```python
from build123d import *

# Parameters (mm, degrees)
PAD_DEPTH       = 18
SKETCH001_R     = 6
POCKET_DEPTH    = 18
SKETCH006_R     = 12.75
POCKET003_DEPTH = 2.4


with BuildPart() as part:
    # Sketch → Pad (new body)
    with BuildSketch(Plane.XY):
        with BuildLine():
            Line((-360, 420), (360, 420))
            Line((360, 420), (360, 36))
            ThreePointArc((324, 0), (349.455844, 10.544156), (360, 36))
            Line((324, 0), (-324, 0))
            ThreePointArc((-360, 36), (-349.455844, 10.544156), (-324, 0))
            Line((-360, 36), (-360, 420))
        make_face()
    extrude(amount=PAD_DEPTH)

    # Sketch001 → Pocket (cut)
    with BuildSketch(Plane.XY.offset(18)):
        with Locations((-85, 125)):
            Circle(SKETCH001_R)
        with Locations((-85, 295)):
            Circle(SKETCH001_R)
        with Locations((85, 295)):
            Circle(SKETCH001_R)
        with Locations((85, 125)):
            Circle(SKETCH001_R)
        with BuildLine():
            ThreePointArc((-274, 253), (-290, 269), (-306, 253))
            Line((-306, 253), (-306, 73))
            ThreePointArc((-306, 73), (-290, 57), (-274, 73))
            Line((-274, 73), (-274, 253))
        make_face()
        with BuildLine():
            ThreePointArc((-136.333333, 253), (-152.333333, 269), (-168.333333, 253))
            Line((-168.333333, 253), (-168.333333, 73))
            ThreePointArc((-168.333333, 73), (-152.333333, 57), (-136.333333, 73))
            Line((-136.333333, 73), (-136.333333, 253))
        make_face()
        with BuildLine():
            ThreePointArc((306, 253), (290, 269), (274, 253))
            Line((274, 73), (274, 253))
            ThreePointArc((274, 73), (290, 57), (306, 73))
            Line((306, 253), (306, 73))
        make_face()
        with BuildLine():
            ThreePointArc((168.333333, 253), (152.333333, 269), (136.333333, 253))
            Line((136.333333, 73), (136.333333, 253))
            ThreePointArc((136.333333, 73), (152.333333, 57), (168.333333, 73))
            Line((168.333333, 253), (168.333333, 73))
        make_face()
        with BuildLine():
            Line((-27, 324), (27, 324))
            ThreePointArc((39, 312), (35.485281, 320.485281), (27, 324))
            Line((39, 312), (39, 148))
            ThreePointArc((27, 136), (35.485281, 139.514719), (39, 148))
            Line((27, 136), (-27, 136))
            ThreePointArc((-39, 148), (-35.485281, 139.514719), (-27, 136))
            Line((-39, 148), (-39, 312))
            ThreePointArc((-27, 324), (-35.485281, 320.485281), (-39, 312))
        make_face()
    extrude(amount=-POCKET_DEPTH, mode=Mode.SUBTRACT)

    # Sketch006 → Pocket003 (cut)
    with BuildSketch(Plane.XY.offset(18)):
        with Locations((-85, 295)):
            Circle(SKETCH006_R)
        with Locations((85, 295)):
            Circle(SKETCH006_R)
        with Locations((-85, 125)):
            Circle(SKETCH006_R)
        with Locations((85, 125)):
            Circle(SKETCH006_R)
    extrude(amount=-POCKET003_DEPTH, mode=Mode.SUBTRACT)


solid = part.part
```
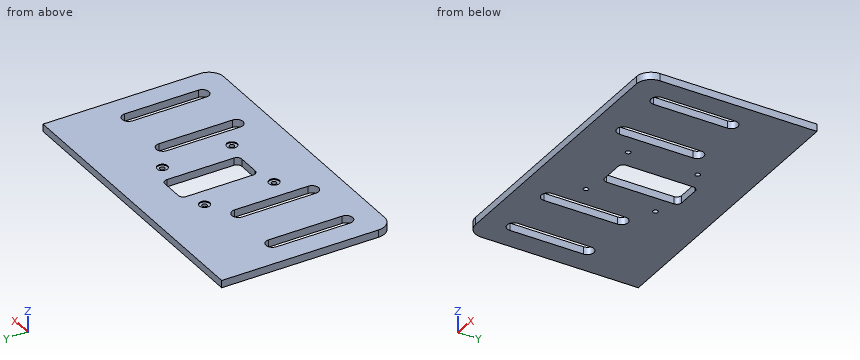
Read the model definition and answer for the solid it produces. Units are mm, in the model's axes. Coordinates: 2 decimals unless noted, no trailing zeros. Write each loop counter-clockwise with the first axis right and the second up, starting at its lowest first coordinate (ties: lowest second). Pieces come first, ordered by that corner, then holes. Notation, with made-up numbers: (49, 67.25) -> (70, 67.25) arc R32 ccw to (70, 96.25) -> close; hole circle Ø2 at (31, 88). An arc over 180 degrees is marked (long way). Return JSON: item names as keys, results as strings.
1. A cutting plane is placed at A-A (y = 182). Determine the outline of the cut face in (x, z), and give its area (3 significant figures).
Found:
{"outline": "(-360, 0) -> (-306, 0) -> (-306, 18) -> (-360, 18) -> close; (-274, 0) -> (-168.33, 0) -> (-168.33, 18) -> (-274, 18) -> close; (-136.33, 0) -> (-39, 0) -> (-39, 18) -> (-136.33, 18) -> close; (39, 0) -> (136.33, 0) -> (136.33, 18) -> (39, 18) -> close; (168.33, 0) -> (274, 0) -> (274, 18) -> (168.33, 18) -> close; (306, 0) -> (360, 0) -> (360, 18) -> (306, 18) -> close", "area": "9,250 mm2"}
2. This flat-tipped pin is pushed along its axis until it touches: P1, Ø7.5, axis at x = 80.5, y = 293, coming from the +Z side. Where does it stop, or does it pass through?
Found:
{"P1": "z = 15.6"}
3. Find the intervals of material crossed by line 1 along X through (y, z) = (207, 4.75); line 2 along Y through (x, z) = (85, 16.55); line 3 along Y through (x, z) = (85, 11.5), in increasing order. Write a range as from..to.
Found:
{"line 1": "-360..-306, -274..-168.33, -136.33..-39, 39..136.33, 168.33..274, 306..360", "line 2": "0..112.25, 137.75..282.25, 307.75..420", "line 3": "0..119, 131..289, 301..420"}
4. A cutting plane is placed at C-C (z = 4.5). Give the number of separate pieces and of enclosed holes in the cut face, and give its area (3 significant figures).
Found:
{"separate pieces": "1", "enclosed holes": "9", "area": "261,000 mm2"}
5. A cutting plane is placed at B-B (y = 82.5). Determine the outline of the cut face in (x, z).
Found:
{"outline": "(-360, 0) -> (-306, 0) -> (-306, 18) -> (-360, 18) -> close; (-274, 0) -> (-168.33, 0) -> (-168.33, 18) -> (-274, 18) -> close; (-136.33, 0) -> (136.33, 0) -> (136.33, 18) -> (-136.33, 18) -> close; (168.33, 0) -> (274, 0) -> (274, 18) -> (168.33, 18) -> close; (306, 0) -> (360, 0) -> (360, 18) -> (306, 18) -> close"}
